The listing builds one solid part. Answer for the finished solid, in the listing's coordinates (mm). A direction names the side the tool comes from. Coordinates: 2 decimals unless noted, no trailing zeros. Loops run counter-clockwise (first coordinate to the right, second up) from the corner with the lowest first, then second, coordinate; pieces in that order, holes last. Notation, with made-up numbers: (-16.5, 14) -> (36.5, 14) arc R4 ccw to (36.5, 20) -> close; hole circle Ø1 at (15.25, -28). An arc over 180 degrees is marked (long way). Answer in a Markdown table with one row per item.
```python
from build123d import *


with BuildPart() as part:
    # Sketch1 → Revolve1 (revolve)
    with BuildSketch(Plane(origin=(0, 0, 0), x_dir=(-1, 0, 0), z_dir=(0, 0, -1))):
        with BuildLine():
            Line((-2.38125, 3.302), (-2.25425, 3.175))
            Line((-2.25425, 3.175), (2.25425, 3.175))
            Line((2.25425, 3.175), (2.38125, 3.302))
            Line((2.38125, 3.302), (2.38125, 3.96875))
            Line((2.38125, 3.96875), (2.00025, 3.96875))
            Line((2.00025, 3.96875), (2.00025, 5.55625))
            Line((2.00025, 5.55625), (2.38125, 5.55625))
            Line((2.38125, 5.55625), (2.38125, 6.111875))
            ThreePointArc((2.38125, 6.111875), (2.311504802, 6.280254802), (2.143125, 6.35))
            Line((2.143125, 6.35), (-2.143125, 6.35))
            ThreePointArc((-2.143125, 6.35), (-2.311504802, 6.280254802), (-2.38125, 6.111875))
            Line((-2.38125, 6.111875), (-2.38125, 5.55625))
            Line((-2.38125, 5.55625), (-2.00025, 5.55625))
            Line((-2.00025, 5.55625), (-2.00025, 3.96875))
            Line((-2.00025, 3.96875), (-2.38125, 3.96875))
            Line((-2.38125, 3.96875), (-2.38125, 3.302))
        make_face()
    revolve(axis=Axis((2.382500003, 0, 0), (-1, 0, 0)))


solid = part.part
```
Item 1: A tool of negligible diameter and unlimited length cuts with its end or side. For faces 5 (the face through (2, -4, -1)), 6 (the face through (-2, 4, -1)), 7 (the face through (2.381, -2, -3)), from which of +Z, -Z, +X, -X, +Y, -Y can it reach the whole face along a straight path? Write none if from no direction.
Findings below:
| item | result |
|---|---|
| face 5 | +X |
| face 6 | -X |
| face 7 | +Z, -Z, +X, +Y, -Y |
Item 2: Find the intervals of material crossed by probe 1 along Z at (x, y) = (2.15, 0) (3 decimals); probe 2 along Y at (x, z) = (0.45, 0) (3 decimals), in increasing order.
Findings below:
| item | result |
|---|---|
| probe 1 | z = -6.35 to -5.556, -3.969 to -3.175, 3.175 to 3.969, 5.556 to 6.35 |
| probe 2 | y = -6.35 to -3.175, 3.175 to 6.35 |
Item 3: Determine the mould class of faces 1 (the face through (-2.19, 5.3, -1.67)), 2 (the face through (2.381, 3, 5)), 3 (the face through (0.03, -1.38, 6.2)), 4 (the face through (-2.188, -0.86, 3.874)) for opening direction Z: +Z half, -Z half, draft (parallel to the pull), parting line (faces both ways), or undercut.
Findings below:
| item | result |
|---|---|
| face 1 | undercut |
| face 2 | draft |
| face 3 | parting line |
| face 4 | undercut |
Item 4: A cutting plane is placed at C-C, the plane x = 0.4. Determine the outline of the cut face in (y, z) (3 decimals), plus the area to 3 significant figures.
Findings below:
| item | result |
|---|---|
| outline | circle Ø12.7 at (0, 0); hole circle Ø6.35 at (0, 0) |
| area | 95.0 mm2 |
Item 5: Flat-ended cylindrical pins translate along their axes: pin 1 Ø2 at (x, y) = (-1.5, -4.5) entering from +Z; pin 2 Ø1 at (x, z) = (2, 1.5) entering from -Y; pin 3 Ø1.5 at (x, z) = (1.5, -2.5) entering from -Y. Find the tip coordinate at first contact, or state that the pin passes through.
Findings below:
| item | result |
|---|---|
| pin 1 | stops at z = 5.3 |
| pin 2 | stops at y = -6.27 |
| pin 3 | stops at y = -6.1 |
